Part model, mm, in its own coordinate system. Coordinates: 2 decimals unless noted, no trailing zeros. Loops run counter-clockwise (first coordinate to the right, second up) from the corner with the lowest first, then second, coordinate; pieces in that order, holes last. Notation, with made-up numbers: M 6.25,-14 L 15.25,-14 A20 ccw 15.25,-6 Z; hole C 60,7 d3. An arc over 180 degrees is marked long. Use a Markdown table: item, result. Add a question column.
1) Band-saw the part on B-B (x = -18.5). List the corners of the cut face in (y, z), plus the area to 3 significant figures.
2) Pin check, flat tips, straight feed: pin 1 Ø6 at (y, z) = (0, 59) entering from -X; pin 2 Ø4.5 at (x, z) = (-3, 48.5) entering from +Y; pin 3 Ø6 at (y, z) = (2, 71.5) entering from -X; pin 4 Ø3 at (x, z) = (-0.02, 49.4) entering from +Y. Stop position of each tip, or through.
3) Wall check: probe 1 along Z at (x, y) = (-1, 2); probe 2 along Y at (x, z) = (-7, 4); probe 3 along Y at (x, z) = (-7, 50). Give the ranges that are in metal, low to high. Write a range as from..to.
4) Band-saw the part on D-D (x = 3). List the corners of the cut face in (y, z).
5) Band-saw the part on A-A (y = 1). List the corners of the cut face in (x, z).
6) Band-saw the part on C-C (z = 55). List the corners of the cut face in (x, y), plus the area to 3 significant figures.
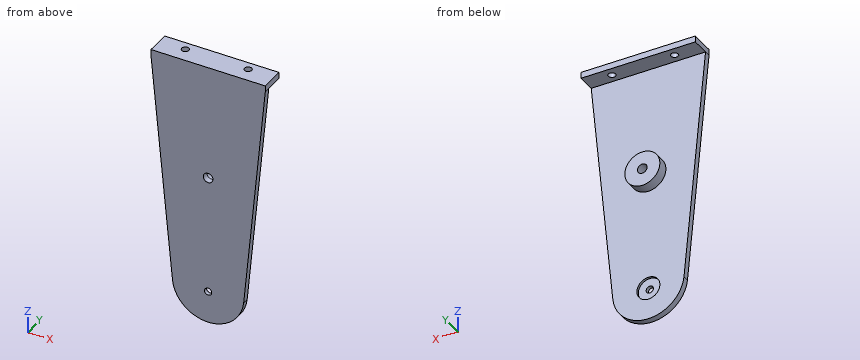
from build123d import *

# Parameters (mm, degrees)
SKETCH2_R           = 1.999999943
BOSS_EXTRUDE3_DEPTH = 2.54
SKETCH3_W           = 47.380920583
SKETCH3_H           = 10
SKETCH3_R           = 1.5
BOSS_EXTRUDE6_DEPTH = 2.54
SKETCH2_5_R         = 1.5
CUT_EXTRUDE1_DEPTH  = 10
SKETCH2_6_R         = 4.7625
SKETCH2_6_R_2       = 1.5
CUT_EXTRUDE2_DEPTH  = 1
SKETCH2_7_R         = 7.267969402
SKETCH2_7_R_2       = 1.999999943
BOSS_EXTRUDE7_DEPTH = 4.420108


with BuildPart() as part:
    # Sketch2 → Boss-Extrude3 (new body)
    with BuildSketch(Plane.XZ):
        with BuildLine():
            Line((14.71851466, 0), (23.68035712, 94.809011723))
            Line((23.68035712, 94.809011723), (-23.700563463, 94.809011723))
            Line((-23.700563463, 94.809011723), (-14.758927346, 0))
            ThreePointArc((-14.758927346, 0), (-0.020206343, -13.282171548), (14.71851466, 0))
        make_face()
        with Locations((-0.020206343, 49.398276345)):
            Circle(SKETCH2_R, mode=Mode.SUBTRACT)
    extrude(amount=BOSS_EXTRUDE3_DEPTH)

    # Sketch3 → Boss-Extrude6 (add)
    with BuildSketch(Plane.XY.offset(94.809011723)):
        with Locations((-0.010103172, 2.46)):
            Rectangle(SKETCH3_W, SKETCH3_H)
        with Locations((-13.010103172, 3.73)):
            Circle(SKETCH3_R, mode=Mode.SUBTRACT)
        with Locations((12.989896828, 3.73)):
            Circle(SKETCH3_R, mode=Mode.SUBTRACT)
    extrude(amount=BOSS_EXTRUDE6_DEPTH)

    # Sketch2<5> → Cut-Extrude1 (cut)
    with BuildSketch(Plane.XZ):
        with Locations((-0.020206343, 0)):
            Circle(SKETCH2_5_R)
    extrude(amount=CUT_EXTRUDE1_DEPTH, mode=Mode.SUBTRACT)

    # Sketch2<6> → Cut-Extrude2 (cut)
    with BuildSketch(Plane.XZ):
        with Locations((-0.020206343, 0)):
            Circle(SKETCH2_6_R)
        with Locations((-0.020206343, 0)):
            Circle(SKETCH2_6_R_2, mode=Mode.SUBTRACT)
    extrude(amount=CUT_EXTRUDE2_DEPTH, mode=Mode.SUBTRACT)

    # Sketch2<7> → Boss-Extrude7 (add)
    with BuildSketch(Plane.XZ):
        with Locations((-0.020206343, 49.398276345)):
            Circle(SKETCH2_7_R)
        with Locations((-0.020206343, 49.398276345)):
            Circle(SKETCH2_7_R_2, mode=Mode.SUBTRACT)
    extrude(amount=-BOSS_EXTRUDE7_DEPTH)


solid = part.part
Entries:
| question | item | result |
|---|---|---|
| 1 | outline | M -2.54,39.67 L 0,39.67 L 0,94.81 L 7.46,94.81 L 7.46,97.35 L -2.54,97.35 Z |
| 1 | area | 165 mm2 |
| 2 | pin 1 | x = -20.61 |
| 2 | pin 2 | y = 4.42 |
| 2 | pin 3 | x = -21.71 |
| 2 | pin 4 | through |
| 3 | probe 1 | 42.2..47.65, 51.14..56.6, 94.81..97.35 |
| 3 | probe 2 | -2.54..0 |
| 3 | probe 3 | -2.54..4.42 |
| 4 | outline | M -2.54,-12.97 L 0,-12.97 L 0,-3.68 L -1,-3.68 L -1,3.68 L 0,3.68 L 0,42.79 L 4.42,42.79 L 4.42,56.01 L 0,56.01 L 0,94.81 L 7.46,94.81 L 7.46,97.35 L -2.54,97.35 Z |
| 5 | outline | M -23.7,94.81 L 23.68,94.81 L 23.68,97.35 L -23.7,97.35 Z; C -0.02,49.4 d14.54; hole C -0.02,49.4 d4 |
| 6 | outline | M -19.95,-2.54 L 19.92,-2.54 L 19.92,0 L 4.61,0 L 4.61,4.42 L -4.65,4.42 L -4.65,0 L -19.95,0 Z |
| 6 | area | 142 mm2 |
